Answer from the drawing. Dimensions are ordinates in mm from the lowest x, y and z of the part. A direction names the side the tool comes from. Coordinates: 2 decimals unless noted, no trailing zeros. Write each loop counter-clockwise with the first axis right and the second up, starting at its lowest first coordinate (ties: lowest second). Pieces come first, ordered by that corner, then holes.
(1) The part is cut by section A-A, the plane z = 1.1. Determine the outline of the cut face in (x, y), and give its area (3 significant figures).
(2) Given pin 1 (0.6 mm diameter, centred on x = 4, z = 4.5, fed in from +Y); pin 2 (0.6 mm diameter, centred on y = 0.5, z = 1.5, fed in from -X), each flat-ended and moving along its own axis, determine where each tip first touches the part or whether it passes through.
(3) The part is cut by section C-C, the plane x = 5.5. Determine the outline of the cut face in (y, z), and give its area (3 significant figures).
(4) The part is cut by section B-B, the plane y = 0.5. Determine the outline of the cut face in (x, z).
(5) Which of the six approach directions +Z, -Z, +X, -X, +Y, -Y give full straight-line access (tool end or side, diameter ignored) to the marked faces 1, 2 and 3?
(6) The part is cut by section D-D, the plane y = 1.1. Determine the outline of the cut face in (x, z).
(7) Straight lines are drawn through the part: line 1 along Z through (x, y) = (5, 0.2); line 2 along X through (y, z) = (1.25, 2.5); line 3 along X through (y, z) = (0.45, 3.6). For each, find the intervals that lie inside material, in ascending order.
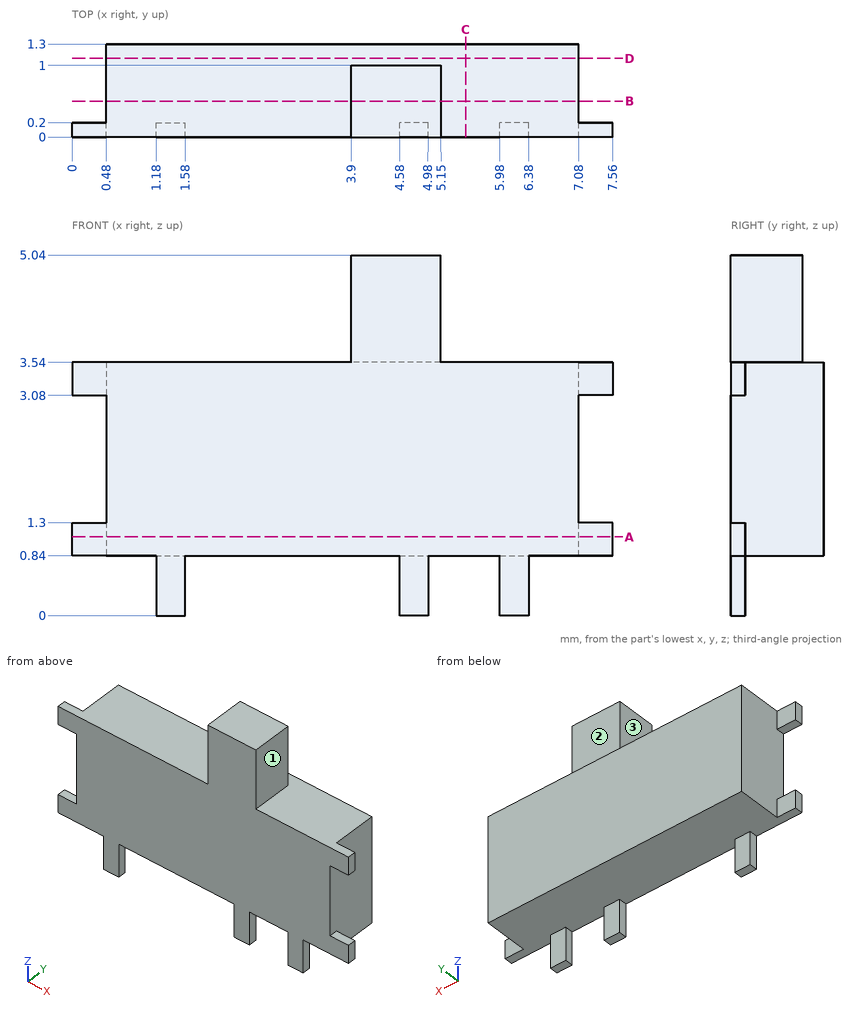
Computed:
1. outline: (0, 0) - (7.56, 0) - (7.56, 0.2) - (7.08, 0.2) - (7.08, 1.3) - (0.48, 1.3) - (0.48, 0.2) - (0, 0.2) - close
1. area: 8.77 mm2
2. pin 1: stops at y = 1
2. pin 2: stops at x = 0.48
3. outline: (0, 0.84) - (1.3, 0.84) - (1.3, 3.54) - (0, 3.54) - close
3. area: 3.51 mm2
4. outline: (0.48, 0.84) - (7.08, 0.84) - (7.08, 3.54) - (5.15, 3.54) - (5.15, 5.04) - (3.9, 5.04) - (3.9, 3.54) - (0.48, 3.54) - close
5. face 1: +Z, +X, +Y, -Y
5. face 2: +Z, +X, -X, +Y
5. face 3: +Z, -X, +Y, -Y
6. outline: (0.48, 0.84) - (7.08, 0.84) - (7.08, 3.54) - (0.48, 3.54) - close
7. line 1: z = 0.84 to 5.04
7. line 2: x = 0.48 to 7.08
7. line 3: x = 3.9 to 5.15
